from build123d import *

# Parameters (mm, degrees)
BOSS_EXTRUDE1_DEPTH     = 7.7
SKETCH2_W               = 7
SKETCH2_H               = 3.1
CUT_EXTRUDE1_DEPTH      = 79.027559234
FILLET1_R               = 10
BOSS_EXTRUDE2_DEPTH     = 2
BOSS_EXTRUDE3_DEPTH     = 33.45
BOSS_EXTRUDE4_REACH     = 112.929
CUT_EXTRUDE2_DEPTH      = 111.928772192
CUT_EXTRUDE2_DEPTH_BACK = 111.928772192
CUT_EXTRUDE3_DEPTH      = 10
FILLET3_R               = 1
FILLET5_R               = 3
CUT_EXTRUDE4_REACH      = 113.176
SKETCH8_W               = 17
SKETCH8_H               = 5
SKETCH8_W_2             = 19
SKETCH8_H_2             = 7
FILLET6_R               = 2
FILLET7_R               = 2


with BuildPart() as part:
    # Sketch1 → Boss-Extrude1 (new body)
    with BuildSketch(Plane(origin=(0, 0, 0), x_dir=(1, 0, 0), z_dir=(0, 1, 0))):
        Polygon((0, 0), (-16.35, 0), (-16.35, -9.85), (-2.6, -9.85), (-2.6, -33), (-20.1, -33), (-20.1, -75), (0, -75), align=None)
    extrude(amount=BOSS_EXTRUDE1_DEPTH)

    # Sketch2 → Cut-Extrude1 (cut, through all)
    with BuildSketch(Plane.XY.offset(75)):
        with Locations((-16.6, 3.55)):
            Rectangle(SKETCH2_W, SKETCH2_H)
    extrude(amount=-CUT_EXTRUDE1_DEPTH, mode=Mode.SUBTRACT)

    # Fillet1
    fillet1_edges = [part.edges().sort_by_distance(p)[0] for p in [
        (-2.6, 3.85, 33),
    ]]
    fillet(fillet1_edges, radius=FILLET1_R)

    # Sketch3 → Boss-Extrude2 (add)
    with BuildSketch(Plane(origin=(0, 7.7, 0), x_dir=(1, 0, 0), z_dir=(0, 1, 0))):
        Polygon((0, 4.5), (-33.45, 4.5), (-33.45, -75), (-10, -105), (0, -105), align=None)
    extrude(amount=BOSS_EXTRUDE2_DEPTH)

    # Sketch4 → Boss-Extrude3 (add)
    with BuildSketch(Plane(origin=(0, 0, 0), x_dir=(0, 0, -1), z_dir=(1, 0, 0))):
        Polygon((-105, 9.7), (-105, 12.7), (-90, 12.7), (-50.25, 9.7), align=None)
    extrude(amount=-BOSS_EXTRUDE3_DEPTH)

    # Boss-Extrude4: up to this face of the body (flat: up to its plane)
    boss_extrude4_end = Plane(part.part.faces().sort_by_distance((0, 5.848980441, 46.191947566))[0])
    # Sketch5 → Boss-Extrude4 (add, up to the picked face)
    with BuildSketch(Plane.ZY.offset(33.45), mode=Mode.PRIVATE) as boss_extrude4_sk1:
        Polygon((75, 7.7), (75, -5), (82, -5), (105, 7.7), align=None)
    boss_extrude4_tool1 = split(extrude(boss_extrude4_sk1.sketch, amount=-BOSS_EXTRUDE4_REACH, mode=Mode.PRIVATE), bisect_by=boss_extrude4_end, keep=Keep.BOTH, mode=Mode.PRIVATE)
    add(boss_extrude4_tool1.solids().sort_by(Axis((-33.45, 2.665766, 85.441441), (1, 0, 0)))[0])

    # Sketch6 → Cut-Extrude2 (cut, two sides: drawn at the far end of the back side and taken through both)
    with BuildSketch(Plane(origin=(0, 7.7, 0), x_dir=(1, 0, 0), z_dir=(0, 1, 0)).offset(-CUT_EXTRUDE2_DEPTH_BACK)):
        Polygon((-33.45, -75), (-10, -105), (-33.45, -105), align=None)
    extrude(amount=CUT_EXTRUDE2_DEPTH + CUT_EXTRUDE2_DEPTH_BACK, mode=Mode.SUBTRACT)

    # Sketch7 → Cut-Extrude3 (cut)
    with BuildSketch(Plane(origin=(0, 0, 0), x_dir=(0, 0, -1), z_dir=(1, 0, 0))):
        Polygon((-75, 0), (-85, 0), (-80, -5), (-75, -5), align=None)
    extrude(amount=-CUT_EXTRUDE3_DEPTH, mode=Mode.SUBTRACT)

    # Fillet3
    # the kernel refuses this fillet: 1 mm, written as the material it takes off along each edge
    with BuildSketch(Plane(origin=(5.810983209, -5, 80), x_dir=(0, 0, 1), z_dir=(-1, 0, 0))) as fillet3_piece_1:
        with BuildLine():
            CenterArc((2.350701034, 0.936487472), FILLET3_R, 135, 114.469800521)
            Line((1.643594253, 1.643594253), (1.629452117, 1.657736389))
            Line((1.629452117, 1.657736389), (-0.014142136, 0.014142136))
            Line((-0.014142136, 0.014142136), (0, -0.02))
            ThreePointArc((0, -0.02), (1, -0.02), (1.992985979, -0.018729749))
            Line((1.992985979, -0.018729749), (2, 0))
        make_face()
    extrude(amount=15.810983209, mode=Mode.SUBTRACT)
    with BuildSketch(Plane(origin=(-10, -5, 82.5), x_dir=(-1, 0, 0), z_dir=(0, 0, -1))) as fillet3_piece_2_section:
        with BuildLine():
            CenterArc((FILLET3_R, FILLET3_R), FILLET3_R, 180, 90)
            Line((0, FILLET3_R), (-FILLET3_R * 0.02, FILLET3_R))
            Line((-FILLET3_R * 0.02, FILLET3_R), (-FILLET3_R * 0.02, -FILLET3_R * 0.02))
            Line((-FILLET3_R * 0.02, -FILLET3_R * 0.02), (FILLET3_R, -FILLET3_R * 0.02))
            Line((FILLET3_R, -FILLET3_R * 0.02), (FILLET3_R, 0))
        make_face()
    fillet3_piece_2 = extrude(amount=10, mode=Mode.PRIVATE)
    fillet3_piece_2 = split(fillet3_piece_2, bisect_by=Plane(origin=(-10.222841489, -6.700692184, 78.299307816), z_dir=(0, 0.7071067811865466, -0.7071067811865485)), keep=Keep.TOP, mode=Mode.PRIVATE)
    add(fillet3_piece_2, mode=Mode.SUBTRACT)
    with BuildSketch(Plane(origin=(5.810983209, -5, 80), x_dir=(0, 0, 1), z_dir=(-1, 0, 0))) as fillet3_piece_3a_section:
        with BuildLine():
            CenterArc((2.350701034, 0.936487472), FILLET3_R, 135, 114.469800521)
            Line((1.643594253, 1.643594253), (1.629452117, 1.657736389))
            Line((1.629452117, 1.657736389), (-0.014142136, 0.014142136))
            Line((-0.014142136, 0.014142136), (0, -0.02))
            ThreePointArc((0, -0.02), (1, -0.02), (1.992985979, -0.018729749))
            Line((1.992985979, -0.018729749), (2, 0))
        make_face()
    fillet3_piece_3a = extrude(amount=21.621966417, mode=Mode.PRIVATE)
    fillet3_piece_3a = split(fillet3_piece_3a, bisect_by=Plane(origin=(-10, -4.567151235, 80.996776665), z_dir=(-1, 0, 0)), keep=Keep.TOP, mode=Mode.PRIVATE)
    with BuildSketch(Plane(origin=(-10, -5, 82.5), x_dir=(-1, 0, 0), z_dir=(0, 0, -1))) as fillet3_piece_3b_section:
        with BuildLine():
            CenterArc((FILLET3_R, FILLET3_R), FILLET3_R, 180, 90)
            Line((0, FILLET3_R), (-FILLET3_R * 0.02, FILLET3_R))
            Line((-FILLET3_R * 0.02, FILLET3_R), (-FILLET3_R * 0.02, -FILLET3_R * 0.02))
            Line((-FILLET3_R * 0.02, -FILLET3_R * 0.02), (FILLET3_R, -FILLET3_R * 0.02))
            Line((FILLET3_R, -FILLET3_R * 0.02), (FILLET3_R, 0))
        make_face()
    fillet3_piece_3b = extrude(amount=10, mode=Mode.PRIVATE)
    fillet3_piece_3b = split(fillet3_piece_3b, bisect_by=Plane(origin=(-10.238471404, -4.220535034, 80.779464966), z_dir=(0, -0.7071067811865466, 0.7071067811865485)), keep=Keep.TOP, mode=Mode.PRIVATE)
    fillet3_piece_3 = fillet3_piece_3a & fillet3_piece_3b
    add(fillet3_piece_3, mode=Mode.SUBTRACT)

    # Mirror1: part across plane


with BuildPart() as part_1:
    add(part.part)
    add(part.part.mirror(Plane(origin=(0, 7.7, 75), x_dir=(0, 0, 1), z_dir=(-1, 0, 0))))

    # Fillet5
    # the kernel refuses this fillet: 3 mm, written as the material it takes off along each edge
    with BuildSketch(Plane(origin=(-38.068859068, -5, 69.091011854), x_dir=(0, 1, 0), z_dir=(0.6158478756904763, 0, 0.7878650861711843)), Plane(origin=(38.068859068, -5, 69.091011854), x_dir=(-0.7878650861711843, 0, -0.6158478756904764), z_dir=(-0.6158478756904763, 0, 0.7878650861711843))) as fillet5_piece_1:
        with BuildLine():
            CenterArc((FILLET5_R, -FILLET5_R), FILLET5_R, 90, 90)
            Line((0, -FILLET5_R), (0, 0))
            Line((0, 0), (FILLET5_R, 0))
        make_face()
    extrude(amount=23.884769896, mode=Mode.SUBTRACT)

    # Cut-Extrude4: up to this face of the body (flat: up to its plane)
    cut_extrude4_end = Plane(part_1.part.faces().sort_by_distance((0, 0, 47.459676899))[0])
    # Sketch8 → Cut-Extrude4 (cut, up to the picked face)
    with BuildSketch(Plane(origin=(0, 9.7, 0), x_dir=(1, 0, 0), z_dir=(0, 1, 0)), mode=Mode.PRIVATE) as cut_extrude4_sk1:
        with Locations((24.95, 2)):
            Rectangle(SKETCH8_W, SKETCH8_H)
    cut_extrude4_tool1 = split(extrude(cut_extrude4_sk1.sketch, amount=-CUT_EXTRUDE4_REACH, mode=Mode.PRIVATE), bisect_by=cut_extrude4_end, keep=Keep.BOTH, mode=Mode.PRIVATE)
    # Sketch8 → Cut-Extrude4 (cut, up to the picked face)
    with BuildSketch(Plane(origin=(0, 9.7, 0), x_dir=(1, 0, 0), z_dir=(0, 1, 0)), mode=Mode.PRIVATE) as cut_extrude4_sk2:
        with Locations((-24.95, 2)):
            Rectangle(SKETCH8_W_2, SKETCH8_H_2)
    cut_extrude4_tool2 = split(extrude(cut_extrude4_sk2.sketch, amount=-CUT_EXTRUDE4_REACH, mode=Mode.PRIVATE), bisect_by=cut_extrude4_end, keep=Keep.BOTH, mode=Mode.PRIVATE)
    add(cut_extrude4_tool1.solids().sort_by(Axis((24.95, 9.7, -2), (0, -1, 0)))[0], mode=Mode.SUBTRACT)
    add(cut_extrude4_tool2.solids().sort_by(Axis((-24.95, 9.7, -2), (0, -1, 0)))[0], mode=Mode.SUBTRACT)

    # Fillet6
    fillet6_edges = [part_1.edges().sort_by_distance(p)[0] for p in [
        (-15.45, 8.7, -4.5),
        (-33.45, 8.7, 1.5),
    ]]
    fillet(fillet6_edges, radius=FILLET6_R)

    # Fillet7
    fillet7_edges = [part_1.edges().sort_by_distance(p)[0] for p in [
        (33.45, 8.7, 0.5),
        (16.45, 8.7, -4.5),
    ]]
    fillet(fillet7_edges, radius=FILLET7_R)


solid = part_1.part
Design review of the part built by this model. Coordinates are the model's own, in mm. A direction names the side the tool comes from. Give positions to 0.01 mm unless a question says otherwise; leave off trailing zeros. Loops run counter-clockwise (first coordinate to the right, second up) from the corner with the lowest first, then second, coordinate; pieces in that order, holes last. Notation, with made-up numbers: M 38.5,46 L 82.5,46 A19 cw 82.5,51 Z; hole C 53.5,12 d6. An arc over 180 degrees is marked long. One line per question, with ' | ' between items. Start each with the question number.
1. Add section B-B (z = 47.5). Write out the cut boundary in (x, y), plus the area to 3 significant figures.
2. Insertion check: P1, Ø1.6, axis at y = 0.5, z = 0.5, coming from the -X side; P2, Ø6, axis at y = 6.5, z = 68, coming from the +X side; P3, Ø2, axis at x = 10.5, y = -2, coming from the -Z side; P4, Ø0.9, axis at y = 3.5, z = 57.5, coming from the +X side. Each pin has a flat end and moves straight along its axis. Give the tip position at first contact, or say it passes through.
3. Add section A-A (z = 11.5). Write out the cut boundary in (x, y).
4. Add section D-D (z = 73.5). Write out the cut boundary in (x, y).
5. To check wall thickness, follow L1, parallel to Y at x = 29, z = 47; L2, parallel to Y at x = -8.5, z = 54.5; L3, parallel to Y at x = 18.5, z = 58. State the ranges of each line that lie inside material, in increasing order.
6. For faces 4 (the face through (-16.35, 6, 6)), 5 (the face through (10, 4, 9.85)), 6 (the face through (13.1, 4, 54)), list the 3-axis set-ups (+Z, -Z, +X, -X, +Y, -Y) from which the entire face can be reached by the end or side of a thin tool; tool diameter is ignored.
7. Add section C-C (z = 28.5). Write out the cut boundary in (x, y), plus the area to 3 significant figures.
8. The part is to be moulded in two halves that separate along Z. For faces 1 (the face through (-16, 6, 33)), 2 (the face through (-13.1, 4, 54)), 3 (the face through (0, 10, 105)), say which applies: released by +Z, released by -Z, zero draft, split by the parting line, or undercut.
Worked out:
1) outline: M -33.45,7.7 L -20.1,7.7 L -20.1,5.1 L -13.1,5.1 L -13.1,2 L -20.1,2 L -20.1,0 L 20.1,0 L 20.1,2 L 13.1,2 L 13.1,5.1 L 20.1,5.1 L 20.1,7.7 L 33.45,7.7 L 33.45,9.7 L -33.45,9.7 Z | area: 400 mm²
2) P1: stops at x = -15.45 | P2: stops at x = 33.45 | P3: stops at z = 75 | P4: stops at x = 13.1
3) outline: M -33.45,7.7 L -2.6,7.7 L -2.6,0 L 2.6,0 L 2.6,7.7 L 33.45,7.7 L 33.45,9.7 L -33.45,9.7 Z
4) outline: M -33.45,7.7 L -20.1,7.7 L -20.1,5.1 L -13.1,5.1 L -13.1,2 L -20.1,2 L -20.1,0 L 20.1,0 L 20.1,2 L 13.1,2 L 13.1,5.1 L 20.1,5.1 L 20.1,7.7 L 33.45,7.7 L 33.45,11.45 L -33.45,11.45 Z
5) L1: y = 7.7 to 9.7 | L2: y = 0 to 10.02 | L3: y = 0 to 2, 5.1 to 10.28
6) face 4: -Z, -X, -Y | face 5: +X, -Y | face 6: -Z, +X
7) outline: M -33.45,7.7 L -4.25,7.7 L -4.25,0 L 4.25,0 L 4.25,7.7 L 33.45,7.7 L 33.45,9.7 L -33.45,9.7 Z | area: 199 mm²
8) face 1: undercut | face 2: zero draft | face 3: released by +Z
